```python
from build123d import *

# Parameters (mm, degrees)
F0_W     = 150
F0_H     = 20
F1_DEPTH = 2
F2_R     = 7
F3_DEPTH = 25
F4_R     = 7
F4_R_2   = 5
F5_DEPTH = 15


with BuildPart() as f1:
    # F0 (on Top) → F1 (new body)
    with BuildSketch(Plane.XY):
        Rectangle(F0_W, F0_H)
    extrude(amount=F1_DEPTH)

    # F2 (on face) → F3 (join)
    with BuildSketch(Plane.XY.offset(2)):
        Circle(F2_R)
    extrude(amount=F3_DEPTH)

    # F4 (on face) → F5 (cut)
    with BuildSketch(Plane.XY.offset(27)):
        Circle(F4_R)
        Circle(F4_R_2, mode=Mode.SUBTRACT)
    extrude(amount=-F5_DEPTH, mode=Mode.SUBTRACT)


solid = f1.part
```
Geometry check sheet. Reference: the model listing, model coordinates, mm. A direction names the side the tool comes from. Give positions to 0.01 mm unless a question says otherwise; leave off trailing zeros. Loops run counter-clockwise (first coordinate to the right, second up) from the corner with the lowest first, then second, coordinate; pieces in that order, holes last. Notation, with made-up numbers: (10, 44) - (23, 44) arc R29 cw to (23, 74) - close; hole circle Ø11 at (18, -25.75). An arc over 180 degrees is marked (long way). Use CSV: the item, a comma, the result in double quotes. Start each with the question number.
Q1. Access from +Z, -Z, +X, -X, +Y, -Y to the whole of each face (thin tool, end or side, straight path). Record for faces 1 (the face through (6.466, -2.681, 6.93)), 2 (the face through (-1, 0, 0)).
Q2. Section check D-D, the plane z = 22. Record the cut outline in (x, y), and give its area (3 significant figures).
Q3. Section check B-B, the plane y = 0. Record the cut outline in (x, z).
Q4. Section check A-A, the plane x = 0. Record the cut outline in (y, z).
Q5. Section check C-C, the plane z = 7. Record the cut outline in (x, y), and give its area (3 significant figures).
Q6. Go/stop test with flat-tipped pins: pin 1 Ø2 at (x, z) = (-3, 14) entering from +Y; pin 2 Ø12 at (y, z) = (0.5, 21) entering from -X; pin 3 Ø1 at (y, z) = (4, 6.5) entering from +X. Record where each tip stops, or that it passes through.
Q7. Scan lines: probe 1 along Z at (x, y) = (-37, 1.5); probe 2 along X at (y, z) = (-1.75, 21.75); probe 3 along X at (y, z) = (4.25, 18). Record each from-to range of solid material in increasing order. Write a range as from..to.
Findings below:
1,face 1,"+Z"
1,face 2,"-Z, +X, -X, +Y, -Y"
2,outline,"circle Ø10 at (0, 0)"
2,area,"78.5 mm^2"
3,outline,"(-75, 0) - (75, 0) - (75, 2) - (7, 2) - (7, 12) - (5, 12) - (5, 27) - (-5, 27) - (-5, 12) - (-7, 12) - (-7, 2) - (-75, 2) - close"
4,outline,"(-10, 0) - (10, 0) - (10, 2) - (7, 2) - (7, 12) - (5, 12) - (5, 27) - (-5, 27) - (-5, 12) - (-7, 12) - (-7, 2) - (-10, 2) - close"
5,outline,"circle Ø14 at (0, 0)"
5,area,"154 mm^2"
6,pin 1,"stops at y = 4.58"
6,pin 2,"stops at x = -5"
6,pin 3,"stops at x = 6.06"
7,probe 1,"z = 0..2"
7,probe 2,"x = -4.68..4.68"
7,probe 3,"x = -2.63..2.63"
